Here's how the part is built. I have some questions about the finished solid (model axes, mm). Give positions to 0.01 mm unless a question says otherwise; leave off trailing zeros. Loops run counter-clockwise (first coordinate to the right, second up) from the corner with the lowest first, then second, coordinate; pieces in that order, holes last. Notation, with made-up numbers: (-5, 52) -> (32, 52) arc R32 ccw to (32, 86) -> close; hole circle Ø11 at (-35.5, -25.5). An arc over 180 degrees is marked (long way). Answer in a Markdown table with one row per item. Add a question column.
Item 1: If I drill on line 1 (Z direction, x = 8.5, y = -138); line 2 (Z direction, x = 11, y = -169), over which ranges is the centre line in solid material (lowest first)?
Item 2: If we section it at A-A (x = 9): Write out the boundary of the cut face in (y, z), then the cut area to 3 significant figures.
Item 3: If we section it at B-B (y = 13): Write out the boundary of the cut face in (x, z), then the cut area to 4 significant figures.
Item 4: For P1, Ø1.5, axis at y = -156, z = 79, coming from the -X side, with a flat end and sliding along its axis, tell me the tip position at first contact or that it passes through.
```python
from build123d import *

# Parameters (mm, degrees)
F0_W     = 480
F0_H     = 360
F1_DEPTH = 12
F3_DEPTH = 480.001
F4_DEPTH = 24


with BuildPart() as f1:
    # F0 (on Right) → F1 (new body)
    with BuildSketch(Plane.YZ):
        Rectangle(F0_W, F0_H)
    extrude(amount=F1_DEPTH)

    # F2 (on face) → F3 (cut, through all)
    with BuildSketch(Plane(origin=(0, 240, 0), x_dir=(-1, 0, 0), z_dir=(0, 1, 0))):
        Polygon((-12, -175), (-12, -180), (-7, -180), align=None)
        Polygon((-7, -60), (-12, -60), (-12, -65), align=None)
        Polygon((-12, -55), (-12, -60), (-7, -60), align=None)
        Polygon((-7, 60), (-12, 60), (-12, 55), align=None)
        Polygon((-12, 65), (-12, 60), (-7, 60), align=None)
        Polygon((-7, 180), (-12, 180), (-12, 175), align=None)
    extrude(amount=-F3_DEPTH, mode=Mode.SUBTRACT)

    # F4 (cut): a face of the model
    f4_faces = [f1.faces().sort_by_distance(p)[0] for p in [
        (5.9234393404, -240, 0),
    ]]
    extrude(f4_faces, amount=-F4_DEPTH, mode=Mode.SUBTRACT)


solid = f1.part
```
Recorded:
| question | item | result |
|---|---|---|
| 1 | line 1 | z = -178.5 to -61.5, -58.5 to 58.5, 61.5 to 178.5 |
| 1 | line 2 | z = -176 to -64, -56 to 56, 64 to 176 |
| 2 | outline | (-216, -178) -> (240, -178) -> (240, -62) -> (-216, -62) -> close; (-216, -58) -> (240, -58) -> (240, 58) -> (-216, 58) -> close; (-216, 62) -> (240, 62) -> (240, 178) -> (-216, 178) -> close |
| 2 | area | 159,000 mm^2 |
| 3 | outline | (0, -180) -> (7, -180) -> (12, -175) -> (12, -65) -> (7, -60) -> (12, -55) -> (12, 55) -> (7, 60) -> (12, 65) -> (12, 175) -> (7, 180) -> (0, 180) -> close |
| 3 | area | 4,245 mm^2 |
| 4 | P1 | stops at x = 0 |
